Answer from the drawing. Dimensions are ordinates in mm from the lowest x, y and z of the part. A direction names the side the tool comes from. Round coordinates to 2 decimals unless told otherwise and drop trailing zeros. Order: outer loops, then holes, each group sorted by start corner. A loop starts at its lowest first (then second) coordinate and runs counter-clockwise, first axis right, second up. Notation, with made-up numbers: M 18,25 L 47,25 A5 cw 47,33 Z; hole C -5.5,60 d1. An arc over 180 degrees is marked long. Answer as a JSON object with one key per item and string values. Group by question number.
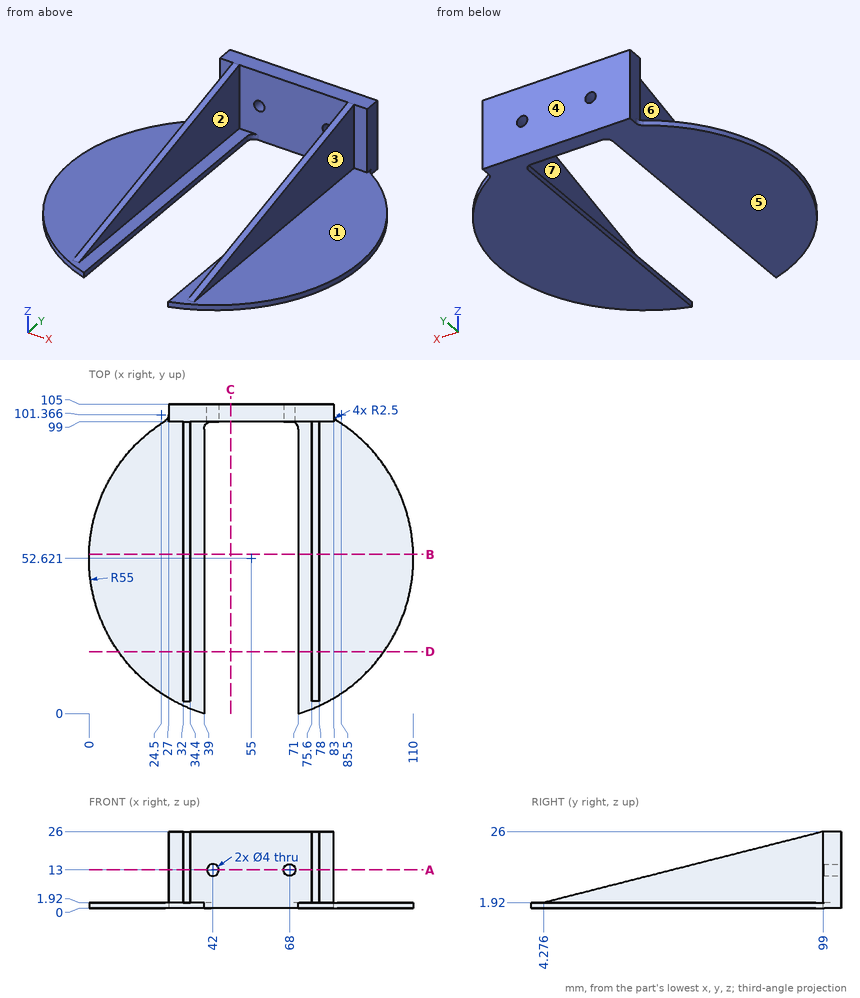
Item 1: Find section C-C (x = 48). Give the vertices of the cut face in (y, z), and give its area (3 significant figures).
Item 2: Each of these flat-tipped pins is pushed along its axis until it touches: pin 1 (0.6 mm diameter, centred on y = 49, z = 1, fed in from -X); pin 2 (4.5 mm diameter, centred on x = 68, z = 13, fed in from +Y); pin 3 (13 mm diameter, centred on x = 57, z = 16, fed in from -Y); pin 4 (2 mm diameter, centred on y = 28.5, z = 4, fed in from -X). Where does it stop, or does it pass through?
Item 3: Find section D-D (y = 21). Give the vertices of the cut face in (x, z), and give its area (3 significant figures).
Item 4: A tool of negligible diameter and unlimited length cuts with its end or side. For the marked faces 5, 6 and 7, from which of +Z, -Z, +X, -X, +Y, -Y can it reach the whole face along a straight path? Write none if from no direction.
Item 5: Find section B-B (y = 54). Give the vertices of the cut face in (x, z).
Item 6: Consider L1, parallel to Z at x = 42, y = 102.8; L2, parallel to Y at x = 70.5, z = 7; L3, parallel to Z at x = 94, y = 63.5. Determine where each line is inside the solid, lowest interval first.
Item 7: The mould has two halves that part along X. Classify the marked faces 1, 2, 3 and 4: +X half, -X half, draft (parallel to the pull), parting line (faces both ways), or undercut.
Item 8: Find section A-A (z = 13). Give the vertices of the cut face in (x, y).
Responses:
{
 "1": {"outline": "M 99,0 L 105,0 L 105,26 L 99,26 Z", "area": "156 mm^2"},
 "2": {"pin 1": "stops at x = 0.1", "pin 2": "stops at y = 105", "pin 3": "stops at y = 99", "pin 4": "stops at x = 32"},
 "3": {"outline": "M 10,0 L 39,0 L 39,1.92 L 34.4,1.92 L 34.4,6.17 L 32,6.17 L 32,1.92 L 10,1.92 Z; M 71,0 L 100,0 L 100,1.92 L 78,1.92 L 78,6.17 L 75.6,6.17 L 75.6,1.92 L 71,1.92 Z", "area": "132 mm^2"},
 "4": {"face 5": "-Z, +X, -X, +Y, -Y", "face 6": "+Z, -X, -Y", "face 7": "+Z, -Y"},
 "5": {"outline": "M 0.02,0 L 39,0 L 39,1.92 L 34.4,1.92 L 34.4,14.56 L 32,14.56 L 32,1.92 L 0.02,1.92 Z; M 71,0 L 109.98,0 L 109.98,1.92 L 78,1.92 L 78,14.56 L 75.6,14.56 L 75.6,1.92 L 71,1.92 Z"},
 "6": {"L1": "z = 0 to 11, 15 to 26", "L2": "y = 99 to 105", "L3": "z = 0 to 1.92"},
 "7": {"face 1": "undercut", "face 2": "undercut", "face 3": "+X half", "face 4": "draft"},
 "8": {"outline": "M 27,99 L 32,99 L 32,47.86 L 34.4,47.86 L 34.4,99 L 40,99 L 40,105 L 27,105 Z; M 44,99 L 66,99 L 66,105 L 44,105 Z; M 70,99 L 75.6,99 L 75.6,47.86 L 78,47.86 L 78,99 L 83,99 L 83,105 L 70,105 Z"}
}
